For this review, take the finished solid that the model builds, in its own axes (mm). Face numbers are marked on the shaded views. Round coordinates to 2 decimals unless told otherwise and drop trailing zeros. Loops run counter-clockwise (first coordinate to the right, second up) from the corner with the lowest first, then second, coordinate; pieces in that order, holes last.
1) Take a section at B-B (z = 9.25). State the section outline as (x, y) points.
2) Mouldability with a two-part tool opening along X and no side actions: class the marked faces 1, 2 and 3 as pulls with the +X half, pulls with the -X half, needs draft (parallel to the pull), parting line crosses it, or undercut.
3) Wall thickness on L1, parallel to X at y = 25, z = -3.25; L2, parallel to Z at x = 44.5, y = 16.25; L3, parallel to Y at x = -15.5, z = 3.25: over which ranges is each line inside the solid? List them lowest first.
4) Insertion check: pin 1 (4 mm diameter, centred on x = -35.5, y = 16.5, fed in from +Z); pin 2 (2 mm diameter, centred on y = 11.5, z = -9.5, fed in from +X); pin 3 (10 mm diameter, centred on x = 54, y = 24, fed in from +Z). Each pin has a flat end and moves straight along its axis. Give the tip position at first contact, or say it passes through.
5) Take a section at C-C (x = 42). State the section outline as (y, z) points, then the cut area to 4 significant figures.
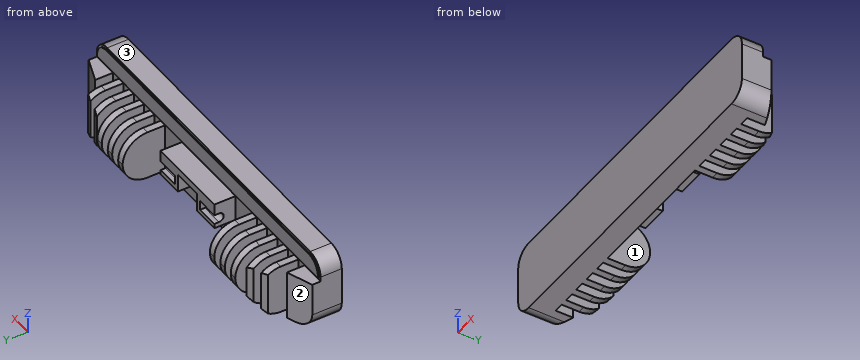
```python
from build123d import *

# Parameters (mm, degrees)
BOSS_EXTRUDE1_DEPTH    = 9
BOSS_EXTRUDE2_DEPTH    = 0.5
SKETCH3_W              = 3
SKETCH3_H              = 21
BOSS_EXTRUDE3_DEPTH    = 7.5
CHAMFER1_SIZE          = 10.75
CHAMFER1_SIZE_2        = 4
CHAMFER2_SIZE          = 4
CHAMFER2_SIZE_2        = 10.75
SKETCH4_W              = 3
SKETCH4_H              = 21
BOSS_EXTRUDE4_DEPTH    = 10.5
FILLET1_R              = 10.5
CUT_EXTRUDE1_START     = 22.980740698
CUT_EXTRUDE1_OUTLINE_W = 3
CUT_EXTRUDE1_OUTLINE_H = 19
CUT_EXTRUDE1_DEPTH     = 4.019259302
CHAMFER3_SIZE2         = 3
CHAMFER3_SIZE          = 1
CUT_EXTRUDE2_START     = 24.646741863
CUT_EXTRUDE2_OUTLINE_W = 3
CUT_EXTRUDE2_OUTLINE_H = 17
CUT_EXTRUDE2_DEPTH     = 2.353258137
CHAMFER4_SIZE2         = 3
CHAMFER4_SIZE          = 1
CUT_EXTRUDE3_START     = 22.980740698
CUT_EXTRUDE3_OUTLINE_W = 3
CUT_EXTRUDE3_OUTLINE_H = 19
CUT_EXTRUDE3_DEPTH     = 4.019259302
CUT_EXTRUDE4_START     = 24.646741863
CUT_EXTRUDE4_OUTLINE_W = 3
CUT_EXTRUDE4_OUTLINE_H = 17
CUT_EXTRUDE4_DEPTH     = 2.353258137
CHAMFER5_SIZE2         = 3
CHAMFER5_SIZE          = 1
CHAMFER6_SIZE2         = 3
CHAMFER6_SIZE          = 1
BOSS_EXTRUDE5_DEPTH    = 9
SKETCH10_W             = 9.5
SKETCH10_H             = 4
CUT_EXTRUDE5_DEPTH     = 4
FILLET2_R              = 2
FILLET3_R              = 2


# Read off the part's stored shape, not the designer's step: Cut-Extrude1, Cut-Extrude2, Cut-Extrude3, Cut-Extrude4
# Some blends are built 0.0001 mm under size
with BuildPart() as part:
    # Sketch1 → Boss-Extrude1 (new body)
    with BuildSketch(Plane(origin=(0, 0, 0), x_dir=(1, 0, 0), z_dir=(0, 1, 0))):
        with BuildLine():
            Line((0, 15), (68, 15))
            ThreePointArc((68, 15), (72.949747468, 12.949747468), (75, 8))
            Line((75, 8), (75, -8))
            ThreePointArc((75, -8), (72.949747468, -12.949747468), (68, -15))
            Line((68, -15), (-68, -15))
            ThreePointArc((-68, -15), (-72.949747468, -12.949747468), (-75, -8))
            Line((-75, -8), (-75, 8))
            ThreePointArc((-75, 8), (-72.949747468, 12.949747468), (-68, 15))
            Line((-68, 15), (0, 15))
        make_face()
    extrude(amount=BOSS_EXTRUDE1_DEPTH)

    # Sketch2 → Boss-Extrude2 (add)
    with BuildSketch(Plane(origin=(0, 9, 0), x_dir=(1, 0, 0), z_dir=(0, 1, 0))):
        with BuildLine():
            Line((74, -7), (-74, -7))
            Line((-74, -7), (-74, -8))
            ThreePointArc((-74, -8), (-72.242640687, -12.242640687), (-68, -14))
            Line((-68, -14), (68, -14))
            ThreePointArc((68, -14), (72.242640687, -12.242640687), (74, -8))
            Line((74, -8), (74, -7))
        make_face()
    extrude(amount=BOSS_EXTRUDE2_DEPTH)

    # Sketch3 → Boss-Extrude3 (add)
    with BuildSketch(Plane(origin=(0, 9, 0), x_dir=(1, 0, 0), z_dir=(0, 1, 0))):
        with BuildLine():
            Line((64.25, -6), (75, -6))
            Line((75, -6), (75, 8))
            ThreePointArc((75, 8), (72.949747468, 12.949747468), (68, 15))
            Line((68, 15), (64.25, 15))
            Line((64.25, 15), (64.25, -6))
        make_face()
        with BuildLine():
            Line((-75, -6), (-64.25, -6))
            Line((-64.25, -6), (-64.25, 15))
            Line((-64.25, 15), (-68, 15))
            ThreePointArc((-68, 15), (-72.949747468, 12.949747468), (-75, 8))
            Line((-75, 8), (-75, -6))
        make_face()
        with Locations((-58.75, 4.5)):
            Rectangle(SKETCH3_W, SKETCH3_H)
        with Locations((-51.75, 4.5)):
            Rectangle(SKETCH3_W, SKETCH3_H)
        with Locations((-44.75, 4.5)):
            Rectangle(SKETCH3_W, SKETCH3_H)
        with Locations((-37.75, 4.5)):
            Rectangle(SKETCH3_W, SKETCH3_H)
        with Locations((-30.75, 4.5)):
            Rectangle(SKETCH3_W, SKETCH3_H)
        with Locations((30.75, 4.5)):
            Rectangle(SKETCH3_W, SKETCH3_H)
        with Locations((37.75, 4.5)):
            Rectangle(SKETCH3_W, SKETCH3_H)
        with Locations((44.75, 4.5)):
            Rectangle(SKETCH3_W, SKETCH3_H)
        with Locations((51.75, 4.5)):
            Rectangle(SKETCH3_W, SKETCH3_H)
        with Locations((58.75, 4.5)):
            Rectangle(SKETCH3_W, SKETCH3_H)
    extrude(amount=BOSS_EXTRUDE3_DEPTH)

    # Chamfer1
    # the kernel refuses this chamfer: 10.75, 4 mm, written as the material it takes off along each edge
    with BuildSketch(Plane(origin=(-75, 16.5, -35.885033622), x_dir=(0.9999096242158825, 0.013444084217698377, 0), z_dir=(0, 0, 1))) as chamfer1_piece_1:
        Polygon((CHAMFER1_SIZE * 0.999909624216, -CHAMFER1_SIZE * 0.0134440842177), (-CHAMFER1_SIZE_2 * 0.0134440842177, -CHAMFER1_SIZE_2 * 0.999909624216), (0, 0), align=None)
    extrude(amount=69.770067243, mode=Mode.SUBTRACT)

    # Chamfer2
    # the kernel refuses this chamfer: 10.75, 4 mm, written as the material it takes off along each edge
    with BuildSketch(Plane(origin=(75, 16.5, 33.885033622), x_dir=(0.09665608708749646, -0.9953178390991163, 0), z_dir=(0, 0, -1))) as chamfer2_piece_1:
        Polygon((CHAMFER2_SIZE * 0.995317839099, CHAMFER2_SIZE * 0.0966560870875), (-CHAMFER2_SIZE_2 * 0.0966560870875, CHAMFER2_SIZE_2 * 0.995317839099), (0, 0), align=None)
    extrude(amount=69.770067243, mode=Mode.SUBTRACT)

    # Sketch4 → Boss-Extrude4 (add)
    with BuildSketch(Plane(origin=(0, 16.5, 0), x_dir=(1, 0, 0), z_dir=(0, 1, 0))):
        with Locations((-44.75, 4.5)):
            Rectangle(SKETCH4_W, SKETCH4_H)
        with Locations((-37.75, 4.5)):
            Rectangle(SKETCH4_W, SKETCH4_H)
        with Locations((-30.75, 4.5)):
            Rectangle(SKETCH4_W, SKETCH4_H)
        with Locations((30.75, 4.5)):
            Rectangle(SKETCH4_W, SKETCH4_H)
        with Locations((37.75, 4.5)):
            Rectangle(SKETCH4_W, SKETCH4_H)
        with Locations((44.75, 4.5)):
            Rectangle(SKETCH4_W, SKETCH4_H)
        with Locations((51.75, 4.5)):
            Rectangle(SKETCH4_W, SKETCH4_H)
        with Locations((58.75, 4.5)):
            Rectangle(SKETCH4_W, SKETCH4_H)
        with Locations((-51.75, 4.5)):
            Rectangle(SKETCH4_W, SKETCH4_H)
        with Locations((-58.75, 4.5)):
            Rectangle(SKETCH4_W, SKETCH4_H)
    extrude(amount=BOSS_EXTRUDE4_DEPTH)

    # Fillet1
    fillet1_edges = [part.edges().sort_by_distance(p)[0] for p in [
        (30.75, 27, 6),
        (37.75, 27, 6),
        (44.75, 27, 6),
        (51.75, 27, 6),
        (58.75, 27, 6),
        (58.75, 27, -15),
        (51.75, 27, -15),
        (44.75, 27, -15),
        (37.75, 27, -15),
        (30.75, 27, -15),
        (-30.75, 27, 6),
        (-37.75, 27, 6),
        (-44.75, 27, 6),
        (-51.75, 27, 6),
        (-58.75, 27, 6),
        (-30.75, 27, -15),
        (-37.75, 27, -15),
        (-44.75, 27, -15),
        (-51.75, 27, -15),
        (-58.75, 27, -15),
    ]]
    fillet(fillet1_edges, radius=FILLET1_R - 0.0001)  # a hair under: the kernel refuses the full size

    # Cut-Extrude1 outline → Cut-Extrude1 (cut)
    with BuildSketch(Plane(origin=(0, 0, 0), x_dir=(1, 0, 0), z_dir=(0, 1, 0)).offset(CUT_EXTRUDE1_START)):
        with Locations((-58.75, 4.5)):
            Rectangle(CUT_EXTRUDE1_OUTLINE_W, CUT_EXTRUDE1_OUTLINE_H)
    extrude(amount=CUT_EXTRUDE1_DEPTH, mode=Mode.SUBTRACT)

    # Chamfer3
    chamfer3_edges = [part.edges().sort_by_distance(p)[0] for p in [
        (-60.25, 22.980740698, -4.5),
    ]]
    chamfer3_side = [part.faces().sort_by_distance(p)[0] for p in [
        (-60.25, 22.960740698, -4.5),
    ]]
    chamfer(chamfer3_edges, length=CHAMFER3_SIZE - 0.0001, length2=CHAMFER3_SIZE2 - 0.0001, reference=chamfer3_side[0])  # a hair under: the kernel refuses the full size

    # Cut-Extrude2 outline → Cut-Extrude2 (cut)
    with BuildSketch(Plane(origin=(0, 0, 0), x_dir=(1, 0, 0), z_dir=(0, 1, 0)).offset(CUT_EXTRUDE2_START)):
        with Locations((-51.75, 4.5)):
            Rectangle(CUT_EXTRUDE2_OUTLINE_W, CUT_EXTRUDE2_OUTLINE_H)
    extrude(amount=CUT_EXTRUDE2_DEPTH, mode=Mode.SUBTRACT)

    # Chamfer4
    chamfer4_edges = [part.edges().sort_by_distance(p)[0] for p in [
        (-53.25, 24.646741863, -4.5),
    ]]
    chamfer4_side = [part.faces().sort_by_distance(p)[0] for p in [
        (-53.25, 24.626741863, -4.5),
    ]]
    chamfer(chamfer4_edges, length=CHAMFER4_SIZE - 0.0001, length2=CHAMFER4_SIZE2 - 0.0001, reference=chamfer4_side[0])  # a hair under: the kernel refuses the full size

    # Cut-Extrude3 outline → Cut-Extrude3 (cut)
    with BuildSketch(Plane(origin=(0, 0, 0), x_dir=(1, 0, 0), z_dir=(0, 1, 0)).offset(CUT_EXTRUDE3_START)):
        with Locations((58.75, 4.5)):
            Rectangle(CUT_EXTRUDE3_OUTLINE_W, CUT_EXTRUDE3_OUTLINE_H)
    extrude(amount=CUT_EXTRUDE3_DEPTH, mode=Mode.SUBTRACT)

    # Cut-Extrude4 outline → Cut-Extrude4 (cut)
    with BuildSketch(Plane(origin=(0, 0, 0), x_dir=(1, 0, 0), z_dir=(0, 1, 0)).offset(CUT_EXTRUDE4_START)):
        with Locations((51.75, 4.5)):
            Rectangle(CUT_EXTRUDE4_OUTLINE_W, CUT_EXTRUDE4_OUTLINE_H)
    extrude(amount=CUT_EXTRUDE4_DEPTH, mode=Mode.SUBTRACT)

    # Chamfer5
    chamfer5_edges = [part.edges().sort_by_distance(p)[0] for p in [
        (60.25, 22.980740698, -4.5),
    ]]
    chamfer5_side = [part.faces().sort_by_distance(p)[0] for p in [
        (60.25, 22.960740698, -4.5),
    ]]
    chamfer(chamfer5_edges, length=CHAMFER5_SIZE - 0.0001, length2=CHAMFER5_SIZE2 - 0.0001, reference=chamfer5_side[0])  # a hair under: the kernel refuses the full size

    # Chamfer6
    chamfer6_edges = [part.edges().sort_by_distance(p)[0] for p in [
        (53.25, 24.646741863, -4.5),
    ]]
    chamfer6_side = [part.faces().sort_by_distance(p)[0] for p in [
        (53.25, 24.626741863, -4.5),
    ]]
    chamfer(chamfer6_edges, length=CHAMFER6_SIZE - 0.0001, length2=CHAMFER6_SIZE2 - 0.0001, reference=chamfer6_side[0])  # a hair under: the kernel refuses the full size

    # Sketch9 → Boss-Extrude5 (add)
    with BuildSketch(Plane(origin=(0, 9, 0), x_dir=(1, 0, 0), z_dir=(0, 1, 0))):
        Polygon((-18, 5), (-6.5, 5), (-6.5, -3), (6.5, -3), (6.5, 5), (18, 5), (18, -6), (-18, -6), align=None)
    extrude(amount=BOSS_EXTRUDE5_DEPTH)

    # Sketch10 → Cut-Extrude5 (cut)
    with BuildSketch(Plane(origin=(0, 18, 0), x_dir=(1, 0, 0), z_dir=(0, 1, 0))):
        with Locations((13.25, 1)):
            Rectangle(SKETCH10_W, SKETCH10_H)
        with Locations((-13.25, 1)):
            Rectangle(SKETCH10_W, SKETCH10_H)
    extrude(amount=-CUT_EXTRUDE5_DEPTH, mode=Mode.SUBTRACT)

    # Fillet2
    fillet2_edges = [part.edges().sort_by_distance(p)[0] for p in [
        (13.25, 14, -3),
        (-13.25, 14, -3),
    ]]
    fillet(fillet2_edges, radius=FILLET2_R)

    # Fillet3
    fillet3_edges = [part.edges().sort_by_distance(p)[0] for p in [
        (-13.25, 14, 1),
        (13.25, 14, 1),
    ]]
    fillet(fillet3_edges, radius=FILLET3_R - 0.0001)  # a hair under: the kernel refuses the full size


solid = part.part
```
Response:
1. outline: (-74.89, 0) - (74.89, 0) - (74.89, 9) - (73.87, 9) - (73.87, 9.5) - (-73.87, 9.5) - (-73.87, 9) - (-74.89, 9) - close
2. face 1: undercut
2. face 2: pulls with the -X half
2. face 3: needs draft
3. L1: x = -46.25 to -43.25, -39.25 to -36.25, -32.25 to -29.25, 29.25 to 32.25, 36.25 to 39.25, 43.25 to 46.25
3. L2: z = -15 to 6
3. L3: y = 0 to 18
4. pin 1: stops at z = 6
4. pin 2: stops at x = 74.98
4. pin 3: stops at z = 5.68
5. outline: (0, -15) - (9, -15) - (9, 7) - (9.5, 7) - (9.5, 14) - (9, 14) - (9, 15) - (0, 15) - close
5. area: 273.5 mm2
